Check sheet for the drawn part. Datum: minimum x, y, z corner. Units: mm. A direction names the side the tool comes from. Give positions to 0.01 mm unless a question says otherwise; leave off trailing zeros. Write each loop counter-clockwise with the first axis right and the second up, starting at its lowest first coordinate (ties: lowest second). Pieces come first, ordered by that corner, then holes.
(1) Mould release check, pull along X, two halves, no side actions. Record for the marked faces 3, 4 and 5: +X half, -X half, draft (parallel to the pull), parting line (faces both ways), or undercut.
(2) Cross-section at D-D (z = 7.5). Record the boundary of the cut face in (x, y).
(3) Cross-section at A-A (x = 7.5). Record the boundary of the cut face in (y, z).
(4) Cross-section at B-B (y = 16.5). Record the boundary of the cut face in (x, z), and give its area (3 significant figures).
(5) Depth check by flat-ended pin: P1, Ø5, axis at y = 10, z = 3.5, coming from the +X side; P2, Ø2.5, axis at x = 6.5, z = 7.5, coming from the +Y side. Enter the tip coordinate at first touch or a pass-through.
(6) Cross-section at C-C (y = 10). Record the boundary of the cut face in (x, z).
(7) Tool access check on the marked faces 1 and 2. Record the directions out of +Z, -Z, +X, -X, +Y, -Y that give a thin tool (end or side, any length) a straight path to the whole face; none if there is none.
(8) Thickness scan on line 1 along X through (y, z) = (4.5, 6); line 2 along X through (y, z) = (17.5, 11.25); line 3 along Z through (x, y) = (3.5, 7). Record the ranges inside material, lowest first.
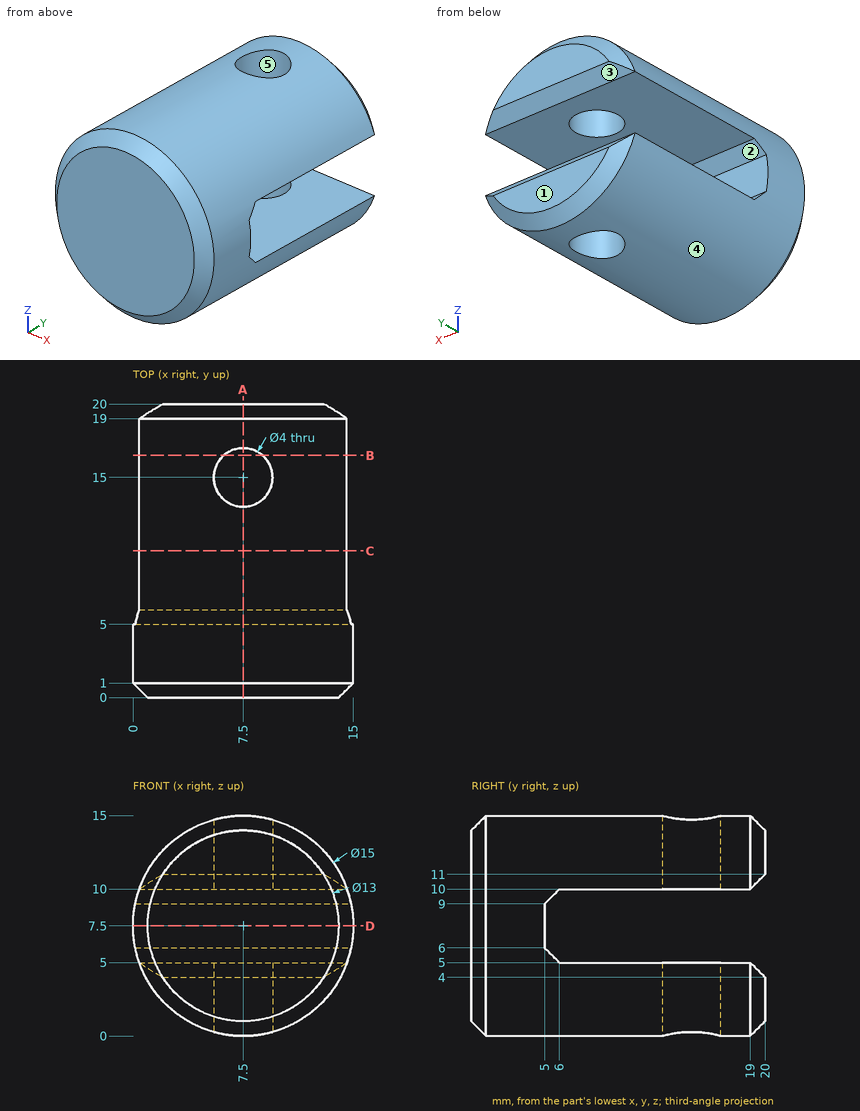
Reply:
1. face 3: draft
1. face 4: parting line
1. face 5: undercut
2. outline: (0, 1) - (1, 0) - (14, 0) - (15, 1) - (15, 5) - (0, 5) - close
3. outline: (0, 1) - (1, 0) - (13, 0) - (13, 5) - (6, 5) - (5, 6) - (5, 9) - (6, 10) - (13, 10) - (13, 15) - (1, 15) - (0, 14) - close; (17, 0) - (19, 0) - (20, 1) - (20, 4) - (19, 5) - (17, 5) - close; (17, 10) - (19, 10) - (20, 11) - (20, 14) - (19, 15) - (17, 15) - close
4. outline: (0.43, 5) arc R7.5 ccw to (6.18, 0.12) - (6.18, 5) - close; (0.43, 10) - (6.18, 10) - (6.18, 14.88) arc R7.5 ccw to start; (8.82, 0.12) arc R7.5 ccw to (14.57, 5) - (8.82, 5) - close; (8.82, 10) - (14.57, 10) arc R7.5 ccw to (8.82, 14.88) - close
4. area: 76.9 mm2
5. P1: stops at x = 14.57
5. P2: stops at y = 5
6. outline: (0.43, 5) arc R7.5 ccw to (14.57, 5) - close; (0.43, 10) - (14.57, 10) arc R7.5 ccw to start
7. face 1: +Z, -Z, +X, -X, +Y
7. face 2: +X, -X, +Y
8. line 1: x = 0.15 to 14.85
8. line 2: x = 1 to 14
8. line 3: z = 1.16 to 5, 10 to 13.84
